Verification items for the finished model (mm, model axes). Face numbers are marked on the shaded views. A direction names the side the tool comes from. Round coordinates to 2 decimals unless told otherwise and drop trailing zeros. Order: outer loops, then holes, each group sorted by start corner. A loop starts at its lowest first (then second) coordinate and runs counter-clockwise, first axis right, second up. Notation, with made-up numbers: (53, -3) -> (71, -3) arc R22 cw to (71, 15) -> close; hole circle Ø7 at (45, -33). An arc over 180 degrees is marked (long way). Return JSON: item names as keys, results as strings. Group by question number.
1) Section check B-B on x = 0. Enter the section's corners in (y, z), plus the area to 3 significant figures.
2) Section check C-C on x = -3. Enter the section's corners in (y, z), plus the area to 3 significant figures.
3) Depth check by flat-ended pin: pin 1 (1 mm diameter, centred on y = 1.5, z = -0.5, fed in from +X). Enter the tip coordinate at first touch or a pass-through.
4) Tool access check on the marked faces 4, 5, 6, 7 and 8. Record the directions out of +Z, -Z, +X, -X, +Y, -Y that give a thin tool (end or side, any length) a straight path to the whole face; none if there is none.
5) Scan lines: L1, parallel to X at y = 1.3, z = 0; L2, parallel to Z at x = 6, y = 0.85; L3, parallel to Z at x = 6.75, y = 0.75. Record each from-to range of solid material in increasing order.
6) Draft check along X on the marked faces 1, 2 and 3. Enter one of: pulls with the +X half, pulls with the -X half, needs draft (parallel to the pull), parting line crosses it, or undercut.
7) Section check D-D on z = -3. Enter the section's corners in (x, y), plus the area to 3 significant figures.
8) Section check A-A on z = 0. Enter the section's corners in (x, y), plus the area to 3 significant figures.
```python
from build123d import *

# Parameters (mm, degrees)
SKETCH1_R           = 8.255
BOSS_EXTRUDE1_DEPTH = 2.3368
SKETCH2_R           = 1.6129
CUT_EXTRUDE1_DEPTH  = 12.905909635
CUT_EXTRUDE6_DEPTH  = 12.905909635
CIRPATTERN1_COUNT   = 20


with BuildPart() as part:
    # Sketch1 → Boss-Extrude1 (new body)
    with BuildSketch(Plane(origin=(0, 0, 0), x_dir=(1, 0, 0), z_dir=(0, 1, 0))):
        with Locations(Location((0, 0, 0), (0, 0, 270))):
            Circle(SKETCH1_R)
    extrude(amount=BOSS_EXTRUDE1_DEPTH)

    # Sketch2 → Cut-Extrude1 (cut, through all)
    with BuildSketch(Plane(origin=(0, 2.3368, 0), x_dir=(1, 0, 0), z_dir=(0, 1, 0))):
        with Locations(Location((0, 0, 0), (0, 0, 270))):
            Circle(SKETCH2_R)
    extrude(amount=-CUT_EXTRUDE1_DEPTH, mode=Mode.SUBTRACT)

    # Sketch3 → Cut-Extrude6 (cut, through all)
    with BuildSketch(Plane(origin=(0, 2.3368, 0), x_dir=(1, 0, 0), z_dir=(0, 1, 0))):
        with BuildLine():
            Line((1.426333388, 8.827371755), (-1.426333388, 8.827371755))
            ThreePointArc((-1.426333388, 8.827371755), (-0.757299678, 7.767926416), (-0.465480831, 6.549373056))
            ThreePointArc((-0.465480831, 6.549373056), (0, 6.565893681), (0.465480831, 6.549373056))
            ThreePointArc((0.465480831, 6.549373056), (0.757299678, 7.767926416), (1.426333388, 8.827371755))
        make_face()
    cut_extrude6 = extrude(amount=-CUT_EXTRUDE6_DEPTH, mode=Mode.SUBTRACT)

    # CirPattern1: Cut-Extrude6 ×20 about axis
    cirpattern1_axis = Axis((0, 0, 0), (0, 1, 0))
    for i in range(1, CIRPATTERN1_COUNT):
        add(cut_extrude6.rotate(cirpattern1_axis, i * 360 / CIRPATTERN1_COUNT), mode=Mode.SUBTRACT)


solid = part.part
```
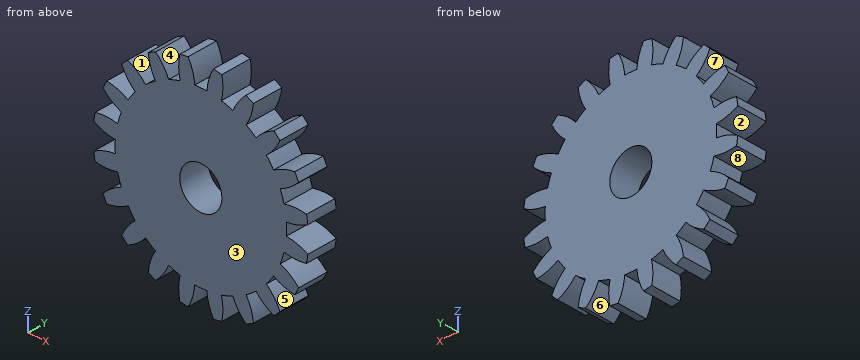
Check result:
{
 "1": {"outline": "(0, -6.57) -> (2.34, -6.57) -> (2.34, -1.61) -> (0, -1.61) -> close; (0, 1.61) -> (2.34, 1.61) -> (2.34, 6.57) -> (0, 6.57) -> close", "area": "23.1 mm^2"},
 "2": {"outline": "(0, -7.01) -> (2.34, -7.01) -> (2.34, 7.01) -> (0, 7.01) -> close", "area": "32.7 mm^2"},
 "3": {"pin 1": "x = 8.2"},
 "4": {"face 4": "+Z, +Y, -Y", "face 5": "+X, +Y, -Y", "face 6": "-Z, +Y, -Y", "face 7": "-X, +Y, -Y", "face 8": "+Y, -Y"},
 "5": {"L1": "-6.57 to -1.61, 1.61 to 6.57", "L2": "-5.67 to -5.47, -3.7 to 3.7, 5.47 to 5.67", "L3": "-3.96 to -2.82, -1.65 to -0.49, 0.49 to 1.65, 2.82 to 3.96"},
 "6": {"face 1": "undercut", "face 2": "pulls with the -X half", "face 3": "needs draft"},
 "7": {"outline": "(-7.01, 0) -> (7.01, 0) -> (7.01, 2.34) -> (-7.01, 2.34) -> close", "area": "32.7 mm^2"},
 "8": {"outline": "(-6.57, 0) -> (-1.61, 0) -> (-1.61, 2.34) -> (-6.57, 2.34) -> close; (1.61, 0) -> (6.57, 0) -> (6.57, 2.34) -> (1.61, 2.34) -> close", "area": "23.1 mm^2"}
}
